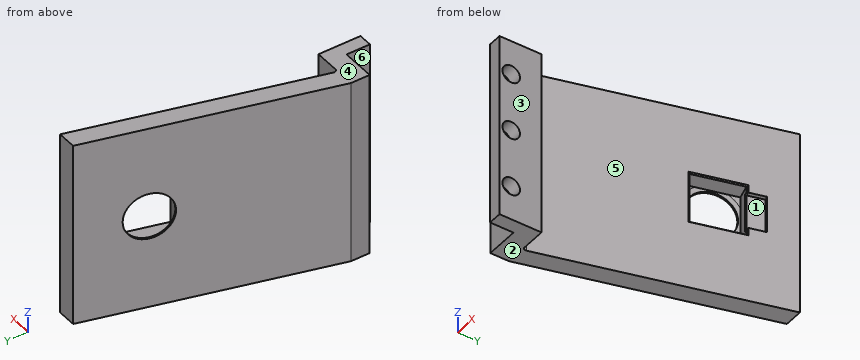
```python
from build123d import *

# Parameters (mm, degrees)
ESQUISSE1_W             = 2.296627968
ESQUISSE1_H             = 4
BOSS_EXTRU_1_DEPTH      = 31.75
ESQUISSE2_W             = 8.53
ESQUISSE2_H             = 8.53
ENL_V_MAT_EXTRU_1_DEPTH = 2.75
ESQUISSE3_R             = 3.98
ENL_V_MAT_EXTRU_2_DEPTH = 31.75
CHANFREIN3_SIZE         = 0.01605866
CHANFREIN3_SIZE_2       = 0.92
ESQUISSE5_W             = 6.3
ESQUISSE5_H             = 3
ENL_V_MAT_EXTRU_3_DEPTH = 0.7
CHANFREIN4_SIZE         = 0.2
ESQUISSE6_R             = 1.5
ENL_V_MAT_EXTRU_4_DEPTH = 14.7
CONG_3_R                = 0.5


with BuildPart() as part:
    # Esquisse1 → Boss.-Extru.1 (new body)
    with BuildSketch(Plane.XY):
        Polygon((3.18, 0), (0, 0), (10.717967697, 40), (13.897967697, 40), align=None)
        Polygon((3.18, 0), (0, 0), (0, -3.18), (5.643372032, -3.18), (7.94, -3.18), (7.94, 0), align=None)
        with Locations((6.791686016, -5.18)):
            Rectangle(ESQUISSE1_W, ESQUISSE1_H)
    extrude(amount=BOSS_EXTRU_1_DEPTH)

    # Esquisse2 → Enlèv. mat.-Extru.1 (cut)
    with BuildSketch(Plane(origin=(2.966980392, -0.795, 0), x_dir=(0, 0, -1), z_dir=(0.9659258262890674, -0.2588190451025244, 0))):
        with Locations((-16.145, 30.088044563)):
            Rectangle(ESQUISSE2_W, ESQUISSE2_H)
    extrude(amount=-ENL_V_MAT_EXTRU_1_DEPTH, mode=Mode.SUBTRACT)

    # Esquisse3 → Enlèv. mat.-Extru.2 (cut)
    with BuildSketch(Plane(origin=(0.31068437, -0.083247626, 0), x_dir=(0, 0, -1), z_dir=(0.9659258262890674, -0.2588190451025245, 0))):
        with Locations(Location((-16.145, 30.055023218, 0), (0, 0, 90))):
            Circle(ESQUISSE3_R)
    extrude(amount=-ENL_V_MAT_EXTRU_2_DEPTH, mode=Mode.SUBTRACT)

    # Chanfrein3
    # the kernel refuses this chamfer: 0.92, 0.01605866 mm, written as the material it takes off along each edge
    with BuildSketch(Plane(origin=(8.08949678, 28.94767551, 16.145), x_dir=(0.2588190451025241, 0.9659258262890673, 0), z_dir=(0, 0, -1))) as chanfrein3_piece_1_section:
        Polygon((3.98, -CHANFREIN3_SIZE * 0.999999983433), (3.98 + CHANFREIN3_SIZE_2, 0), (3.98, 0), align=None)
    chanfrein3_piece_1 = revolve(axis=Axis((8.08949678, 28.94767551, 16.145), (0.9659258262890674, -0.2588190451025245, 0)), mode=Mode.PRIVATE)
    chanfrein3_piece_1 = split(chanfrein3_piece_1, bisect_by=Plane(origin=(9.196219069, 33.100769288, 19.703208658), z_dir=(-0.25881904510252435, -0.9659258262890673, 0)), keep=Keep.TOP, mode=Mode.PRIVATE)
    chanfrein3_piece_1 = split(chanfrein3_piece_1, bisect_by=Plane(origin=(8.615509723, 30.933532505, 20.41), z_dir=(0, 0, -1)), keep=Keep.TOP, mode=Mode.PRIVATE)
    chanfrein3_piece_1 = split(chanfrein3_piece_1, bisect_by=Plane(origin=(8.615509723, 30.933532505, 11.88), z_dir=(0, 0, 1)), keep=Keep.TOP, mode=Mode.PRIVATE)
    chanfrein3_piece_1 = split(chanfrein3_piece_1, bisect_by=Plane(origin=(6.988492614, 24.86142199, 19.703208658), z_dir=(0.25881904510252435, 0.9659258262890673, 0)), keep=Keep.TOP, mode=Mode.PRIVATE)
    add(chanfrein3_piece_1, mode=Mode.SUBTRACT)

    # Esquisse5 → Enlèv. mat.-Extru.3 (cut)
    with BuildSketch(Plane(origin=(2.966980392, -0.795, 0), x_dir=(0, 0, -1), z_dir=(0.9659258262890674, -0.2588190451025244, 0))):
        with Locations((-16.14, 35.853044563)):
            Rectangle(ESQUISSE5_W, ESQUISSE5_H)
    extrude(amount=-ENL_V_MAT_EXTRU_3_DEPTH, mode=Mode.SUBTRACT)

    # Chanfrein4
    chanfrein4_edges = [part.edges().sort_by_distance(p)[0] for p in [
        (10.754339355, 28.267819306, 20.41),
        (9.650476128, 24.148145657, 16.145),
        (10.754339355, 28.267819306, 11.88),
        (11.858202582, 32.387492955, 12.435),
        (11.858202582, 32.387492955, 19.85),
        (11.520128543, 32.478079621, 19.29),
        (11.182054504, 32.568666287, 16.14),
        (11.520128543, 32.478079621, 12.99),
    ]]
    chamfer(chanfrein4_edges, length=CHANFREIN4_SIZE)

    # Esquisse6 → Enlèv. mat.-Extru.4 (cut)
    with BuildSketch(Plane(origin=(7.94, 0, 0), x_dir=(0, 0, -1), z_dir=(1, 0, 0))):
        with Locations(Location((-25.875, -5.18, 0), (0, 0, 90))):
            Circle(ESQUISSE6_R)
        with Locations(Location((-15.875, -5.18, 0), (0, 0, 90))):
            Circle(ESQUISSE6_R)
        with Locations(Location((-5.875, -5.18, 0), (0, 0, 90))):
            Circle(ESQUISSE6_R)
    extrude(amount=-ENL_V_MAT_EXTRU_4_DEPTH, mode=Mode.SUBTRACT)

    # Congé3
    cong_3_edges = [part.edges().sort_by_distance(p)[0] for p in [
        (3.18, 0, 15.875),
    ]]
    fillet(cong_3_edges, radius=CONG_3_R)


solid = part.part
```
Read the model definition and answer for the solid it produces. Units are mm, in the model's axes. Face numbers are marked on the shaded views. A direction names the side the tool comes from. Coordinates: 2 decimals unless noted, no trailing zeros. Write each loop counter-clockwise with the first axis right and the second up, starting at its lowest first coordinate (ties: lowest second). Pieces come first, ordered by that corner, then holes. Notation, with made-up numbers: (-29, -31.5) - (-21, -31.5) arc R29 ccw to (-21, -10.5) - close; hole circle Ø2 at (68.25, -10.75). An arc over 180 degrees is marked (long way). Answer as a JSON object with one key per item and string values. Group by question number.
1. A cutting plane is placed at B-B (z = 5). Determine the outline of the cut face in (x, y).
2. A cutting plane is placed at A-A (y = -5.18). Determine the outline of the cut face in (x, z) (3 decimals).
3. Consider L1, parallel to Z at x = 7.05, y = -5.18 (3 decimals); L2, parallel to X at y = -4, z = 19; L3, parallel to X at y = 21, z = 9. Determine where each line is inside the solid, lowest interval first. Write a range as [from, to].
4. Which of the six approach directions +Z, -Z, +X, -X, +Y, -Y give full straight-line access (tool end or side, diameter ignored) to the marked faces 4, 5 and 6?
5. The mould has two halves that part along Z. Classify the marked faces 1, 2 and 3: +Z half, -Z half, draft (parallel to the pull), parting line (faces both ways), or undercut.
6. A cutting plane is placed at C-C (y = 14). Determine the outline of the cut face in (x, z).
7. Each of these flat-tipped pins is pushed along its axis until it touches: P1, Ø4.5, axis at y = -6, z = 23, coming from the -X side; P2, Ø10, axis at y = 30.5, z = 5.5, coming from the +X side; P3, Ø2.5, axis at y = -5.18, z = 5.875, coming from the -X side; P4, Ø8, axis at y = -3, z = 17, coming from the +X side. Where does it stop, or does it pass through?
Worked out:
{
 "1": {"outline": "(0, -3.18) - (5.64, -3.18) - (5.64, -3.96) - (7.94, -3.96) - (7.94, 0) - (3.83, 0) arc R0.5 cw to (3.35, 0.63) - (13.9, 40) - (10.72, 40) - (0, 0) - close; (5.64, -7.18) - (7.94, -7.18) - (7.94, -6.4) - (5.64, -6.4) - close"},
 "2": {"outline": "(5.643, 0) - (7.94, 0) - (7.94, 4.375) - (5.643, 4.375) - close; (5.643, 7.375) - (7.94, 7.375) - (7.94, 14.375) - (5.643, 14.375) - close; (5.643, 17.375) - (7.94, 17.375) - (7.94, 24.375) - (5.643, 24.375) - close; (5.643, 27.375) - (7.94, 27.375) - (7.94, 31.75) - (5.643, 31.75) - close"},
 "3": {"L1": "z = [0, 4.375], [7.375, 14.375], [17.375, 24.375], [27.375, 31.75]", "L2": "x = [5.64, 7.94]", "L3": "x = [5.63, 8.81]"},
 "4": {"face 4": "+Z, +X, -X, +Y, -Y", "face 5": "+Z, -Z, +X", "face 6": "+Z, -Z, -X, -Y"},
 "5": {"face 1": "undercut", "face 2": "-Z half", "face 3": "draft"},
 "6": {"outline": "(3.75, 0) - (6.93, 0) - (6.93, 31.75) - (3.75, 31.75) - close"},
 "7": {"P1": "stops at x = 5.64", "P2": "stops at x = 12.69", "P3": "passes through", "P4": "stops at x = 7.94"}
}
